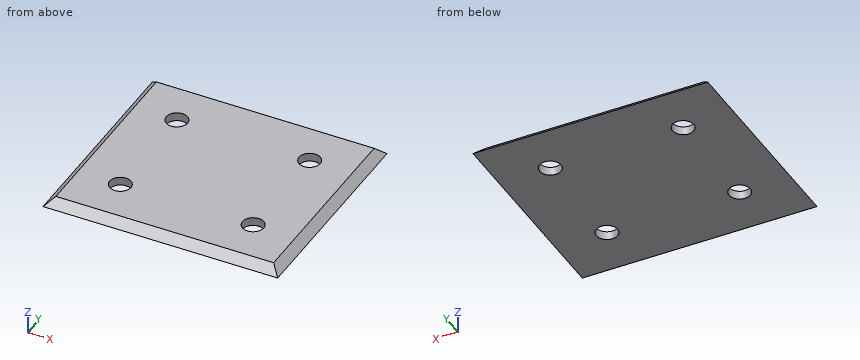
from build123d import *

# Parameters (mm, degrees)
F0_W        = 61.2471848726
F0_H        = 55.7258352637
F1_DEPTH    = 2
F4_D        = 5
F5_T1_DEPTH = 81.4426651434
F5_T3_DEPTH = 86.9640147523


# Not quite as in the source:
# - a fillet or chamfer that OpenCascade refuses, or shapes differently, is made with other operations: its cross-section is extruded or revolved along the edge and cut away or added


with BuildPart() as f1:
    # F0 (on Top) → F1 (new body)
    with BuildSketch(Plane.XY):
        with Locations((30.6235924363, 27.8629176319)):
            Rectangle(F0_W, F0_H)
    extrude(amount=F1_DEPTH)

    # F4 (through all)
    with Locations(Plane(origin=(0, 0, 0), x_dir=(1, 0, 0), z_dir=(0, 0, -1))):
        with Locations((15, -40.7258352637), (46.2471848726, -40.7258352637), (15, -15), (46.2471848726, -15)):
            Hole(F4_D / 2)

    # F5: chamfer of 5 on 4 edges, made by hand

    # F5_s2 → F5_t1 (cut)
    with BuildSketch(Plane.XZ.offset(-68.5842502036)):
        Polygon((0, -3), (5, 2), (0, 2), align=None)
        Polygon((56.2471848726, 2), (61.2471848726, -3), (61.2471848726, 2), align=None)
    extrude(amount=F5_T1_DEPTH, mode=Mode.SUBTRACT)

    # F5_s4 → F5_t3 (cut)
    with BuildSketch(Plane.YZ.offset(-12.8584149398)):
        Polygon((55.7258352637, -3), (50.7258352637, 2), (55.7258352637, 2), align=None)
        Polygon((0, -3), (5, 2), (0, 2), align=None)
    extrude(amount=F5_T3_DEPTH, mode=Mode.SUBTRACT)


solid = f1.part
The listing builds one solid part. Answer for the finished solid, in the listing's coordinates (mm). Give positions to 0.01 mm unless a question says otherwise; leave off trailing zeros. Write each loop counter-clockwise with the first axis right and the second up, starting at its lowest first coordinate (ties: lowest second). Pieces come first, ordered by that corner, then holes.
1) Given P1, Ø4, axis at x = 46.25, y = 40.73, coming from the -Z side; P2, Ø1, axis at y = 23.5, z = 1.5, coming from the +X side, each flat-ended and moving along its own axis, determine where each tip first touches the part or whether it passes through.
2) Section B-B (x = 15) is taken. Write down the section's boundary in (y, z).
3) Section C-C (z = 1.55) is taken. Write down the section's boundary in (x, y), and give its area (3 significant figures).
4) Section A-A (y = 15) is taken. Write down the section's boundary in (x, z).
5) Find the intervals of material crossed by L1, parallel to X at y = 15, z = 0.5; L2, parallel to X at y = 38.5, z = 1.95; L3, parallel to Y at x = 46.5, z = 1.65, in increasing order.
6) Section D-D (y = 30) is taken. Write down the section's boundary in (x, z).
Response:
1. P1: passes through
1. P2: stops at x = 57.25
2. outline: (3, 0) - (12.5, 0) - (12.5, 2) - (5, 2) - close; (17.5, 0) - (38.23, 0) - (38.23, 2) - (17.5, 2) - close; (43.23, 0) - (52.73, 0) - (50.73, 2) - (43.23, 2) - close
3. outline: (4.55, 4.55) - (56.7, 4.55) - (56.7, 51.18) - (4.55, 51.18) - close; hole circle Ø5 at (15, 15); hole circle Ø5 at (15, 40.73); hole circle Ø5 at (46.25, 15); hole circle Ø5 at (46.25, 40.73)
3. area: 2,350 mm2
4. outline: (3, 0) - (12.5, 0) - (12.5, 2) - (5, 2) - close; (17.5, 0) - (43.75, 0) - (43.75, 2) - (17.5, 2) - close; (48.75, 0) - (58.25, 0) - (56.25, 2) - (48.75, 2) - close
5. L1: x = 3.5 to 12.5, 17.5 to 43.75, 48.75 to 57.75
5. L2: x = 4.95 to 13.86, 16.14 to 45.11, 47.39 to 56.3
5. L3: y = 4.65 to 12.51, 17.49 to 38.24, 43.21 to 51.08
6. outline: (3, 0) - (58.25, 0) - (56.25, 2) - (5, 2) - close
